```python
from build123d import *

# Parameters (mm, degrees)
SKETCH1_R                = 2.5
BOSS_EXTRUDE1_DEPTH      = 2
BOSS_EXTRUDE3_DEPTH      = 8
BOSS_EXTRUDE3_DEPTH_BACK = 8
SKETCH3_R                = 5
SKETCH3_R_2              = 2.5


with BuildPart() as part:
    # Sketch1 → Boss-Extrude1 (new body)
    with BuildSketch(Plane(origin=(0, 0, 0), x_dir=(1, 0, 0), z_dir=(0, 1, 0))):
        with BuildLine():
            Line((0, 5), (50, 5))
            ThreePointArc((50, 5), (55, 0), (50, -5))
            Line((50, -5), (0, -5))
            ThreePointArc((0, -5), (-5, 0), (0, 5))
        make_face()
        with Locations(Location((0, 0, 0), (0, 0, 270))):
            Circle(SKETCH1_R, mode=Mode.SUBTRACT)
        with Locations(Location((50, 0, 0), (0, 0, 270))):
            Circle(SKETCH1_R, mode=Mode.SUBTRACT)
    extrude(amount=BOSS_EXTRUDE1_DEPTH)

    # Sketch3 → Boss-Extrude3 (add, two sides: drawn at the far end of the back side and taken through both)
    with BuildSketch(Plane(origin=(0, 1, 0), x_dir=(1, 0, 0), z_dir=(0, 1, 0)).offset(-BOSS_EXTRUDE3_DEPTH_BACK)):
        with Locations(Location((50, 0, 0), (0, 0, 270))):
            Circle(SKETCH3_R)
        with Locations(Location((50, 0, 0), (0, 0, 270))):
            Circle(SKETCH3_R_2, mode=Mode.SUBTRACT)
    extrude(amount=BOSS_EXTRUDE3_DEPTH + BOSS_EXTRUDE3_DEPTH_BACK)


solid = part.part
```
Could you check a few things on this model? Use its own coordinates, in mm. A direction names the side the tool comes from. Coordinates: 2 decimals unless noted, no trailing zeros. Write each loop counter-clockwise with the first axis right and the second up, starting at its lowest first coordinate (ties: lowest second). Pieces come first, ordered by that corner, then holes. Notation, with made-up numbers: (-8, 10.25) - (42, 10.25) arc R24 ccw to (42, 38.25) - close; hole circle Ø9 at (56.5, 12.5). An arc over 180 degrees is marked (long way). Use a Markdown table: item, result.
Q1. Imagine slicing it at D-D (y = 3.75). List the corners of the cut face in (x, z) for me.
Geometry check:
| item | result |
|---|---|
| outline | circle Ø10 at (50, 0); hole circle Ø5 at (50, 0) |
Q2. Imagine slicing it at C-C (x = 49). List the corners of the cut face in (y, z) for me.
Geometry check:
| item | result |
|---|---|
| outline | (-7, -4.9) - (0, -4.9) - (0, -5) - (2, -5) - (2, -4.9) - (9, -4.9) - (9, -2.29) - (-7, -2.29) - close; (-7, 2.29) - (9, 2.29) - (9, 4.9) - (2, 4.9) - (2, 5) - (0, 5) - (0, 4.9) - (-7, 4.9) - close |
Q3. Please list where these lines run through material, in increasing order: L1, parallel to X at y = 1.75, z = 0; L2, parallel to X at y = -3.25, z = 0; L3, parallel to Y at x = 8, z = -3.5.
Geometry check:
| item | result |
|---|---|
| L1 | x = -5 to -2.5, 2.5 to 47.5, 52.5 to 55 |
| L2 | x = 45 to 47.5, 52.5 to 55 |
| L3 | y = 0 to 2 |
Q4. I'm going to push flat-ended pins straight in: pin 1 Ø2 at (x, z) = (16.5, 2) entering from -Y; pin 2 Ø1.5 at (y, z) = (4, 2) entering from +X; pin 3 Ø5 at (y, z) = (5.5, 2.5) entering from -X. Where does each tip first touch, or does it pass through?
Geometry check:
| item | result |
|---|---|
| pin 1 | stops at y = 0 |
| pin 2 | stops at x = 54.84 |
| pin 3 | stops at x = 45 |
Q5. Thinking about a two-plate mould opening in Z: for faces 3 (the cylindrical face through (47.56, 0.89, -0.54)), 4 (the flat face through (25, 1, -5)), 5 (the cylindrical face through (-5, 1, 0)), which applies, +Z half, -Z half, draft (parallel to the pull), parting line (faces both ways), or undercut?
Geometry check:
| item | result |
|---|---|
| face 3 | undercut |
| face 4 | -Z half |
| face 5 | parting line |
Q6. Imagine slicing it at A-A (z = 0). List the corners of the cut face in (x, y) for me, and give its area (3 significant figures).
Geometry check:
| item | result |
|---|---|
| outline | (-5, 0) - (-2.5, 0) - (-2.5, 2) - (-5, 2) - close; (2.5, 0) - (45, 0) - (45, -7) - (47.5, -7) - (47.5, 9) - (45, 9) - (45, 2) - (2.5, 2) - close; (52.5, -7) - (55, -7) - (55, 9) - (52.5, 9) - close |
| area | 170 mm2 |
Q7. Imagine slicing it at B-B (z = -4). List the corners of the cut face in (x, y) for me, and give its area (3 significant figures).
Geometry check:
| item | result |
|---|---|
| outline | (-3, 0) - (47, 0) - (47, -7) - (53, -7) - (53, 9) - (47, 9) - (47, 2) - (-3, 2) - close |
| area | 196 mm2 |
Q8. Which directions (+Z, -Z, +X, -X, +Y, -Y) give clear straight access to the entire face, cutting with the end or side of a thin tool? Please do faces 1 (the flat face through (48, -7, 2)), 2 (the cylindrical face through (54.957, 0.888, -0.651)).
Geometry check:
| item | result |
|---|---|
| face 1 | +Z, -Z, +X, -X, -Y |
| face 2 | none |
